from build123d import *


with BuildPart() as part:
    # Skizze1 → Rotation1 (revolve)
    with BuildSketch(Plane.XY, mode=Mode.PRIVATE) as rotation1_sk:
        Polygon((3.482134942, -20), (13.482134942, -20), (13.482134942, -18), (33.482134942, -18), (33.482134942, -12), (105.482134942, -12), (108.482134942, -15), (108.482134942, -18), (88.482134942, -18), (88.482134942, -20), (38.482134942, -20), (38.482134942, -30), (8.482134942, -30), (8.482134942, -24), (3.482134942, -24), align=None)
    revolve(rotation1_sk.sketch.rotate(Axis((0, 0, 0), (1, 0, 0)), 270), axis=Axis((0, 0, 0), (1, 0, 0)))


solid = part.part
Geometry: final body of the model. Coordinates: model frame, mm. A direction names the side the tool comes from. Round coordinates to 2 decimals unless told otherwise and drop trailing zeros. Order: outer loops, then holes, each group sorted by start corner. A loop starts at its lowest first (then second) coordinate and runs counter-clockwise, first axis right, second up.
Q1. Material intervals for probe 1 along Y at (x, z) = (10, 0); probe 2 along Y at (x, z) = (5, 0); probe 3 along X at (y, z) = (-10, 21), sorted ascending.
Result sheet:
probe 1: y = -30 to -20, 20 to 30
probe 2: y = -24 to -20, 20 to 24
probe 3: x = 3.48 to 38.48
Q2. Pin query (flat end, axial travel): pin 1 (5 mm diameter, centred on x = 72, y = 13.5, fed in from -Z); pin 2 (2 mm diameter, centred on y = 22, z = -19.5, fed in from -X); pin 3 (18 mm diameter, centred on y = -2, z = 3.5, fed in from -X). Return the tip coordinate at first contact, or that it passes through.
Result sheet:
pin 1: stops at z = -16.7
pin 2: stops at x = 8.48
pin 3: stops at x = 33.48
Q3. Section D-D, the plane z = 26. Output: boundary loops of the cut face in (x, y).
Result sheet:
outline: (8.48, -14.97) - (38.48, -14.97) - (38.48, 14.97) - (8.48, 14.97) - close
Q4. Section C-C, the plane x = 79. Output: boundary loops of the cut face in (y, z), and give its area (3 significant figures).
Result sheet:
outline: circle Ø40 at (0, 0); hole circle Ø24 at (0, 0)
area: 804 mm2
Q5. Access query for faces 5 (the face through (88.482, -3, 18)), 6 (the face through (8.482, -20.1, -13.5)), 7 (the face through (23.27, -1.32, -29.97)). Directions: +Z, -Z, +X, -X, +Y, -Y. A direction counts if a zero-diameter tool reaches every point of the face in a straight line with its end or side. Return the directions, or none.
Result sheet:
face 5: +X
face 6: -X
face 7: +X, -X
Q6. Mould query, pull axis Y, two halves, no side actions, for faces 1 (the face through (105.67, -3.661, 11.625)), 2 (the face through (63.132, 19.524, -4.336)), 3 (the face through (3.482, -20, -5)), 4 (the face through (33.482, 12, 4)). Classes: released by +Y, released by -Y, zero draft, split by the parting line, or undercut.
Result sheet:
face 1: undercut
face 2: split by the parting line
face 3: zero draft
face 4: undercut
